Autodesk Inventor part; units mm, degrees
ref_plane "YZ Plane" through (0, 0, 0) normal (1, 0, 0) x (0, 1, 0)
ref_plane "XZ Plane" through (0, 0, 0) normal (0, 1, 0) x (-1, 0, 0)
ref_plane "XY Plane" through (0, 0, 0) normal (0, 0, 1) x (1, 0, 0)
sketch "Эскиз2" plane through (0, 0, 0) normal (0, 1, 0) x (-1, 0, 0)
  line L0 (19, -4) -> (-19, -4)
  line L1 (-19, -4) -> (-19, 4)
  line L2 (-19, 4) -> (19, 4)
  line L3 (19, 4) -> (19, -4)
  line L4 (19, -4) -> (-19, 4) construction
  line L5 (-19, -4) -> (19, 4) construction
  line L6 (19, 0) -> (-19, 0) construction
  circle A0 centre (-15, 0) radius 2
  line L7 (0, -4) -> (0, 4) construction
  circle A1 centre (15, 0) radius 2
  point P0 (0, 0)
  dimension "d1" = 30
  dimension "d2" = 4
  dimension "d3" = 38
  dimension "d4" = 8
extrude "Выдавливание1" add sketch "Эскиз2" along normal blind 35 contours L0 L1 L2 L3 | A0 | A1
fillet "Сопряжение1" radius 3.5 4 edges at (19, 17.5, 4) (19, 17.5, -4) (-19, 17.5, 4) (-19, 17.5, -4)
sketch "Эскиз3" plane through (-15.5, 0, 4) normal (0, 0, 1) x (1, 0, 0)
  line L0 (0, 0) -> (0, 35) construction
  line L1 (0, 0) -> (31, 0) construction
  line L2 (31, 35) -> (31, 0) construction
  line L3 (0, 35) -> (31, 35) construction
  line L4 (34.5, 35) -> (31, 35) construction
  line L5 (31, 35) -> (31, 0) construction
  line L6 (31, 0) -> (34.5, 0) construction
  line L7 (34.5, 0) -> (34.5, 35) construction
  line L8 (0, 35) -> (-3.5, 35) construction
  line L9 (-3.5, 35) -> (-3.5, 0) construction
  line L10 (-3.5, 0) -> (0, 0) construction
  line L11 (0, 0) -> (0, 35) construction
  line L12 (0, 0) -> (0, 35) construction
  line L13 (29, 35) -> (32, 35) construction
  line L14 (29, 0) -> (32, 0) construction
  line L15 (-1, 35) -> (2, 35) construction
  line L16 (-1, 0) -> (2, 0) construction
  line L17 (-1, 35) -> (2, 35) construction
  line L18 (-1, 0) -> (2, 0) construction
  line L19 (29, 35) -> (2, 0) construction
  line L20 (0, 35) -> (31, 35) construction
  line L21 (-3.5, 35) -> (0, 35)
  line L22 (0, 0) -> (31, 0)
  line L23 (0, 35) -> (31, 0) construction
  line L24 (15.5, 17.5) -> (15.5, 0) construction
  circle A0 centre (15.5, 12) radius 10.75
  dimension "d22" = 21.5
  dimension "d23" = 12
extrude "Выдавливание2" cut sketch "Эскиз3" against normal blind 35
sketch "Эскиз4" plane through (-15.5, 0, 4) normal (0, 0, 1) x (1, 0, 0)
  circle A0 centre (15.5, 12) radius 10.5 construction
  line L0 (0, 0) -> (0, 35) construction
  line L1 (0, 0) -> (31, 0) construction
  line L2 (31, 35) -> (31, 0) construction
  line L3 (0, 35) -> (31, 35) construction
  line L4 (0, 35) -> (-3.5, 35) construction
  line L5 (-3.5, 35) -> (-3.5, 0) construction
  line L6 (-3.5, 0) -> (0, 0) construction
  line L7 (0, 0) -> (0, 35) construction
  line L8 (34.5, 35) -> (31, 35) construction
  line L9 (31, 35) -> (31, 0) construction
  line L10 (31, 0) -> (34.5, 0) construction
  line L11 (34.5, 0) -> (34.5, 35) construction
  arc A1 (-1, 2.5793) -> (34.5, 12) centre (15.5, 12) ccw construction
  line L12 (-3.5, 0) -> (-3.5, 35) construction
  line L13 (34.5, 0) -> (34.5, 35) construction
  arc A2 (-3.5, 12) -> (-1, 2.5793) centre (15.5, 12) ccw construction
  line L14 (23.5012, 38.5457) -> (37.6912, 39.4976)
  line L15 (37.6912, 39.4976) -> (34.5, 5)
  circle A3 centre (15.5, 12) radius 15.5
  line L16 (34.5, 0) -> (31, 0) construction
  line L17 (34.5, 0) -> (34.5, 5) construction
  line L18 (34.5, 5) -> (23.6848, 35)
  line L19 (31, 35) -> (0, 35) construction
  line L20 (23.5012, 38.5457) -> (23.6848, 35)
  point P0 (15.5, 0)
  dimension "d18" = 5
  dimension "d24" = 31
extrude "Выдавливание3" cut sketch "Эскиз4" against normal blind 35 contours L14 L15 L18 L20
sketch "Эскиз5" plane through (0, 0, 0) normal (0, -1, 0) x (1, 0, 0)
  circle A0 centre (-15, 0) radius 2
  circle A1 centre (15, 0) radius 2
  point P0 (0, 0)
extrude "Выдавливание4" cut sketch "Эскиз5" against normal up to surface (35 mm away) contours A0
extrude "Выдавливание5" cut sketch "Эскиз5" against normal blind 10 contours A1
fillet "Сопряжение2" radius 0.5 14 edges at (-17.9749, 35, 2.9749) (-19, 35, 0) (-17.9749, 35, -2.9749) (-3.6576, 35, -4) (-3.6576, 35, 4) (8.1848, 35, 0) (17.9749, 0, 2.9749) (19, 0, 0) (17.9749, 0, -2.9749) (0, 0, -4) (-17.9749, 0, -2.9749) (-19, 0, 0) (-17.9749, 0, 2.9749) (0, 0, 4)
ref_plane "РабПлоскость1" through (-18.5, 35, 0) normal (0.3391, -0.9407, 0) x (0.9407, 0.3391, 0)
sketch "Эскиз6" plane through (-18.5, 35, 0) normal (0.3391, -0.9407, 0) x (0.9407, 0.3391, 0)
  ellipse E0 centre (23.0361, 0) end of major axis (23.0361, -2) minor radius 1.8815 construction
  ellipse E1 centre (19.6447, 0) end of major axis (19.6447, -2) minor radius 1.8815 construction
  line L0 (19.6447, 0) -> (23.0361, 0) construction
  circle A0 centre (27.2937, 0) radius 3.5
  point P0 (5.5337, 0)
  dimension "d26" = 7
extrude "Выдавливание6" cut sketch "Эскиз6" along normal blind 20
properties part number "mid_mount_v3" material "Пластик АБС"
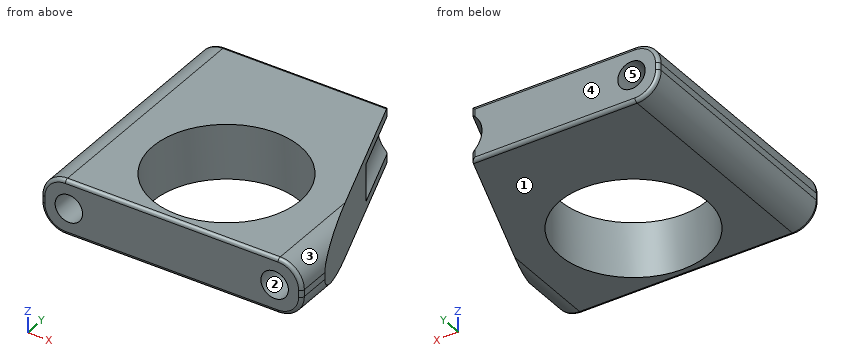
Read the model definition and answer for the solid it produces. Units are mm, in the model's axes. Face numbers are marked on the shaded views. A direction names the side the tool comes from. Give positions to 0.01 mm unless a question says otherwise; leave off trailing zeros. Write each loop counter-clockwise with the first axis right and the second up, starting at its lowest first coordinate (ties: lowest second). Pieces come first, ordered by that corner, then holes. Notation, with made-up numbers: (-16, 12) - (-2, 12) arc R9 ccw to (-2, 23) - close; hole circle Ø5 at (83, 71). An arc over 180 degrees is marked (long way). Use CSV: the item, a comma, the result in double quotes. Start each with the question number.
Item 1: The mould has two halves that part along Z. Classify the marked faces 3, 4 and 5: pulls with the +Z half, pulls with the -Z half, needs draft (parallel to the pull), parting line crosses it, or undercut.
Item 2: A flat-ended cylindrical pin translates along its axis: P1, Ø2.5, axis at x = -15, z = 0, coming from the -Y side. Find the tip coordinate at first contact, or state that the pin passes through.
Item 3: Consider line 1 (Z direction, x = -15, y = 24); line 2 (Y direction, x = 0, z = 1.75); line 3 (X direction, y = 28.5, z = 1.5). Determine where each line is inside the solid, lowest interval first.
Item 4: For the marked faces 1 and 2, determine the directions among +Z, -Z, +X, -X, +Y, -Y from which every point of the face is accessible in a straight line to the end or side of a thin tool.
Item 5: The part is cut by section B-B, the plane x = -15. Give the vertices of the cut face in (y, z).
Item 6: The part is cut by section D-D, the plane x = 14.5. Give the vertices of the cut face in (y, z), and give its area (3 significant figures).
Item 7: The part is cut by section A-A, the plane z = 0. Give the vertices of the cut face in (x, y).
Item 8: The part is cut by section C-C, the plane y = 11. Give the vertices of the cut face in (x, z), and give its area (3 significant figures).
Taken from the geometry:
1,face 3,"pulls with the +Z half"
1,face 4,"needs draft"
1,face 5,"undercut"
2,P1,"through"
3,line 1,"-4 to -2, 2 to 4"
3,line 2,"0 to 1.25, 22.75 to 35"
3,line 3,"-18.85 to -16.32, -13.68 to 9.49"
4,face 1,"-Z, +X, -X, +Y, -Y"
4,face 2,"-Y"
5,outline,"(0, -3.5) arc R0.5 ccw to (0.5, -4) - (34.5, -4) arc R0.5 ccw to (35, -3.5) - (35, -2) - (0, -2) - close; (0, 2) - (35, 2) - (35, 3.5) arc R0.5 ccw to (34.5, 4) - (0.5, 4) arc R0.5 ccw to (0, 3.5) - close"
6,outline,"(0, -3.5) arc R0.5 ccw to (0.5, -4) - (17.48, -4) - (17.48, 4) - (0.5, 4) arc R0.5 ccw to (0, 3.5) - (0, 1.94) - (10, 1.94) - (10, -1.94) - (0, -1.94) - close"
6,area,"101 mm2"
7,outline,"(-19, 0.5) arc R0.5 ccw to (-18.5, 0) - (-17, 0) - (-17, 35) - (-18.5, 35) arc R0.5 ccw to (-19, 34.5) - close; (-13, 0) - (13, 0) - (13, 10) - (17, 10) - (17, 0) - (18.5, 0) arc R0.5 ccw to (19, 0.5) - (19, 5) - (11.9, 24.7) - (10.67, 24.25) - (6.79, 35) - (-13, 35) - close; hole circle Ø21.5 at (0, 12)"
8,outline,"(-19, -0.5) arc R3.5 ccw to (-15.5, -4) - (-10.7, -4) - (-10.7, 4) - (-15.5, 4) arc R3.5 ccw to (-19, 0.5) - close; (10.7, -4) - (15.5, -4) arc R3.5 ccw to (16.84, -3.73) - (16.84, 3.73) arc R3.5 ccw to (15.5, 4) - (10.7, 4) - close; hole circle Ø4 at (-15, 0)"
8,area,"97.4 mm2"
